The model under review builds one solid part; all positions refer to its coordinate system, in mm. Coordinates: 2 decimals unless noted, no trailing zeros. Use one line per item in the form item = value.
from build123d import *

# Parameters (mm, degrees)
SKETCH_2_R               = 3.25
EXTRUDE_1_DEPTH          = 150
CUT_EXTRUDE_START        = -5.375917787
CUT_EXTRUDE_1_DEPTH      = 10.820362331
CUT_EXTRUDE_2_DEPTH      = 178.636263262
CUT_EXTRUDE_2_DEPTH_BACK = 178.636263262
SKETCH_5_R               = 1.75
CUT_EXTRUDE_3_DEPTH      = 154.889291752
FILLET_1_R               = 4
CUT_EXTRUDE_4_DEPTH      = 164.486604715
CUT_EXTRUDE_4_DEPTH_BACK = 164.486604715
SKETCH_8_W               = 10
SKETCH_8_H               = 20
CUT_EXTRUDE_5_DEPTH      = 164.486604715
CUT_EXTRUDE_5_DEPTH_BACK = 164.486604715
SKETCH_9_W               = 3.4
SKETCH_9_H               = 10


# Read off the part's stored shape, not the designer's step: 除料-伸長1
with BuildPart() as part:
    # 草圖2 → 填料-伸長1 (new body)
    with BuildSketch(Plane.XY):
        with BuildLine():
            add(Edge.make_bspline(
                [(-4.885261194, 10), (0, 40), (5, 10)],
                knots=[0, 0, 0, 1, 1, 1], degree=2))
            add(Edge.make_bspline(
                [(5, 10), (7, -20), (0, -95)],
                knots=[0, 0, 0, 1, 1, 1], degree=2))
            add(Edge.make_bspline(
                [(-4.885261194, 10), (-7, -20), (0, -95)],
                knots=[0, 0, 0, 1, 1, 1], degree=2))
        make_face()
        with Locations((0, 5)):
            Circle(SKETCH_2_R, mode=Mode.SUBTRACT)
        with Locations((0, -15)):
            Circle(SKETCH_2_R, mode=Mode.SUBTRACT)
    extrude(amount=EXTRUDE_1_DEPTH)

    # 除料-伸長1 outline → 除料-伸長1 (cut)
    with BuildSketch(Plane(origin=(0, 0, 0), x_dir=(0, 0, -1), z_dir=(1, 0, 0)).offset(CUT_EXTRUDE_START)):
        with BuildLine():
            Line((-150, 25), (-150, -80.493578612))
            add(Edge.make_bspline(
                [(-45.078048967, 25), (-92.099367892, 5.715924734), (-132.413995221, -32.343019704), (-150, -80.493578612)],
                knots=[0, 0, 0, 0, 1, 1, 1, 1], degree=3))
            Line((-45.078048967, 25), (-150, 25))
        make_face()
    extrude(amount=CUT_EXTRUDE_1_DEPTH, mode=Mode.SUBTRACT)

    # 草圖4 → 除料-伸長2 (cut, two sides: drawn at the far end of the back side and taken through both)
    with BuildSketch(Plane(origin=(0, 0, 0), x_dir=(0, 0, -1), z_dir=(1, 0, 0)).offset(-CUT_EXTRUDE_2_DEPTH_BACK)):
        with BuildLine():
            Line((-12, -95), (-12, -45))
            Line((-12, -45), (-105.048136882, -45))
            add(Edge.make_bspline(
                [(-105.048136882, -45), (-130.619727744, -62.828669631), (-133, -95)],
                knots=[0, 0, 0, 1, 1, 1], degree=2))
            Line((-133, -95), (-202.799866115, -110.736264896))
            Line((-202.799866115, -110.736264896), (-206.293444292, 4.551814945))
            Line((-206.293444292, 4.551814945), (-122.032968562, 45.937279504))
            Line((-122.032968562, 45.937279504), (-2.049657297, 49.573137421))
            Line((-2.049657297, 49.573137421), (77.223861612, 25.244547225))
            Line((77.223861612, 25.244547225), (93.885542148, -58.870065807))
            Line((93.885542148, -58.870065807), (27.807345311, -110.736264896))
            Line((27.807345311, -110.736264896), (-12, -95))
        make_face()
    extrude(amount=CUT_EXTRUDE_2_DEPTH + CUT_EXTRUDE_2_DEPTH_BACK, mode=Mode.SUBTRACT)

    # 草圖5 → 除料-伸長3 (cut, through all)
    with BuildSketch(Plane(origin=(0, 0, 12), x_dir=(-1, 0, 0), z_dir=(0, 0, -1))):
        with Locations(Location((0, -55, 0), (0, 0, 90))):
            Circle(SKETCH_5_R)
    extrude(amount=-CUT_EXTRUDE_3_DEPTH, mode=Mode.SUBTRACT)

    # 圓角1
    # the kernel refuses this fillet: 4 mm, written as the material it takes off along each edge
    with BuildSketch(Plane(origin=(-3.97305147, -45, 115.722141015), x_dir=(0.06337202796258917, -0.9979899729315466, 0), z_dir=(0, 0, -1))) as fillet_1_piece_1:
        with BuildLine():
            CenterArc((4.262054506, -3.99999288), FILLET_1_R, 89.891895008, 93.74148946)
            Line((0.270094614, -4.253480992), (0, 0))
            ThreePointArc((0, 0), (2.134800854, 0.002041927), (4.269601653, 0))
        make_face()
    extrude(amount=114.396145149, mode=Mode.SUBTRACT)
    with BuildSketch(Plane(origin=(3.989244513, -45, 115.729130337), x_dir=(-0.06406540579517839, -0.9979457018196427, 0), z_dir=(0, 0, -1))) as fillet_1_piece_2:
        with BuildLine():
            CenterArc((4.265022816, 3.999993202), FILLET_1_R, 176.326807013, 93.77882592)
            Line((0.273240009, 4.256254825), (0, 0))
            ThreePointArc((0, 0), (2.136198717, -0.001996553), (4.272397382, 0))
        make_face()
    extrude(amount=114.410123792, mode=Mode.SUBTRACT)

    # 草圖8 → 除料-伸長4 (cut, two sides: drawn at the far end of the back side and taken through both)
    with BuildSketch(Plane(origin=(0, 0, 0), x_dir=(0, 0, -1), z_dir=(1, 0, 0)).offset(-CUT_EXTRUDE_4_DEPTH_BACK)):
        with Locations((-27, -55.009980051)):
            Rectangle(SKETCH_8_W, SKETCH_8_H)
        with Locations((-109.062447802, -55.009980051)):
            Rectangle(SKETCH_8_W, SKETCH_8_H)
    extrude(amount=CUT_EXTRUDE_4_DEPTH + CUT_EXTRUDE_4_DEPTH_BACK, mode=Mode.SUBTRACT)

    # 草圖9 → 除料-伸長5 (cut, two sides: drawn at the far end of the back side and taken through both)
    with BuildSketch(Plane(origin=(0, 0, 0), x_dir=(0, 0, -1), z_dir=(1, 0, 0)).offset(-CUT_EXTRUDE_5_DEPTH_BACK)):
        with Locations((-38.78, -55)):
            Rectangle(SKETCH_9_W, SKETCH_9_H)
    extrude(amount=CUT_EXTRUDE_5_DEPTH + CUT_EXTRUDE_5_DEPTH_BACK, mode=Mode.SUBTRACT)


solid = part.part
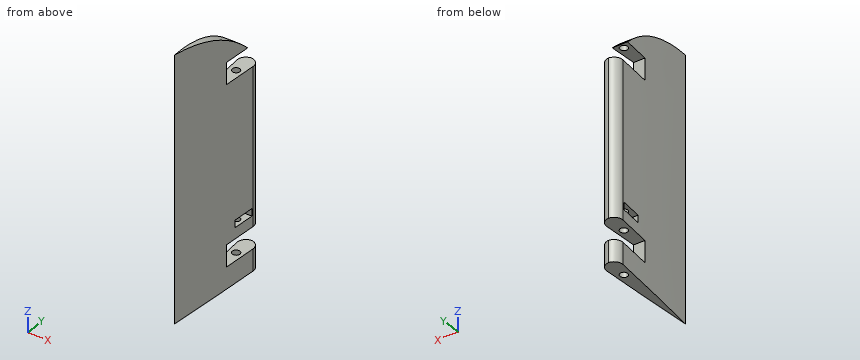
Item 1: Clearance check with flat-ended pins moving along their axes: pin 1 (2.5 mm diameter, centred on x = -1, z = 39.5, fed in from -Y); pin 2 (1 mm diameter, centred on y = -89, z = 73, fed in from -X); pin 3 (2 mm diameter, centred on x = -2, y = -60, fed in from +Z). State where each tip first meets the part, or that it passes through.
Results found:
pin_1 = -95
pin_2 = -0.6
pin_3 = 121.4
Item 2: To check wall thickness, follow L1, parallel to Z at x = 1, y = -51; L2, parallel to Z at x = 2, y = -48; L3, parallel to X at y = -55, z = 69. State the ranges of each line that lie inside material, in increasing order. Write a range as from..to.
Results found:
L1 = 12..22, 32..37.08, 40.48..104.06
L2 = 12..22, 32..104.06
L3 = -3.31..-1.75, 1.75..3.32
Item 3: We need section A-A (y = -55). State how many separate pieces and enclosed holes the cut face has, plus the area to 3 significant figures.
Results found:
separate_pieces = 8
enclosed_holes = 0
area = 255 mm²
